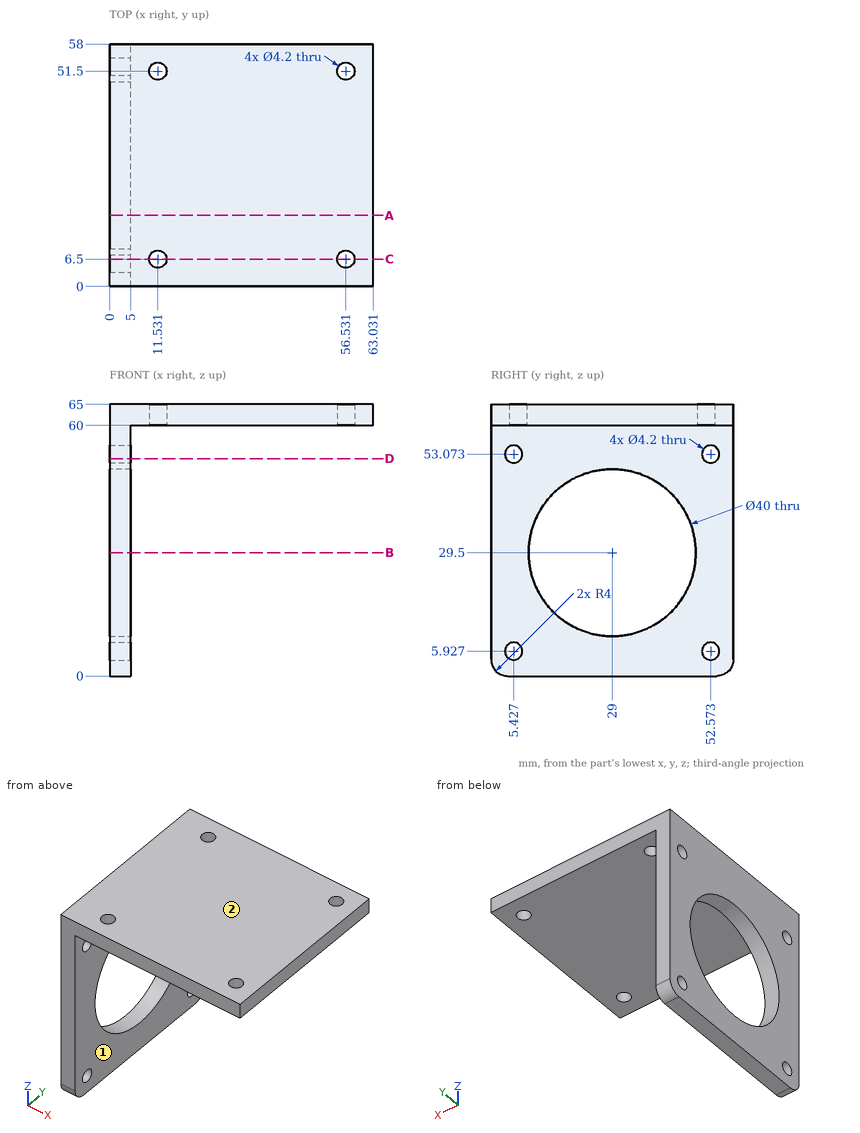
Verification items for this drawing (mm, ordinates from the low corner). A direction names the side the tool comes from. Round coordinates to 2 decimals unless told otherwise and drop trailing zeros. Write each loop counter-clockwise with the first axis right and the second up, starting at its lowest first coordinate (ties: lowest second). Pieces come first, ordered by that corner, then holes. Notation, with made-up numbers: M 24,65 L 50,65 A17 ccw 50,85 Z; hole C 76.25,60 d1. An arc over 180 degrees is marked long. Write item = value, one per line. Start each with the question number.
1. Section check D-D, the plane z = 52. Record the cut outline in (x, y), then the cut area to 3 significant figures.
2. Section check A-A, the plane y = 17. Record the cut outline in (x, z).
3. Section check B-B, the plane z = 29.5. Record the cut outline in (x, y), then the cut area to 3 significant figures.
4. Gauge pin test, flat ends, axial feed: pin 1 (2.5 mm diameter, centred on x = 56.53, y = 51.5, fed in from -Z); pin 2 (5.5 mm diameter, centred on x = 11.53, y = 51.5, fed in from -Z); pin 3 (1 mm diameter, centred on y = 16.5, z = 11, fed in from +X); pin 4 (5 mm diameter, centred on y = 5.43, z = 5.93, fed in from -X). Record the tip position at first contact, or that the pin passes through.
5. Section check C-C, the plane y = 6.5. Record the cut outline in (x, z), then the cut area to 3 significant figures.
6. Scan lines: line 1 (Z direction, x = 46, y = 31.5); line 2 (X direction, y = 18.5, z = 53); line 3 (Z direction, x = 2, y = 29). Record each from-to range of solid material in increasing order. Write a range as [from, to].
7. Tool access check on the marked faces 1 and 2. Record the directions out of +Z, -Z, +X, -X, +Y, -Y that give a thin tool (end or side, any length) a straight path to the whole face; none if there is none.
Results found:
q1.outline = M 0,0 L 5,0 L 5,3.62 L 0,3.62 Z; M 0,7.23 L 5,7.23 L 5,50.77 L 0,50.77 Z; M 0,54.38 L 5,54.38 L 5,58 L 0,58 Z
q1.area = 254 mm^2
q2.outline = M 0,0 L 5,0 L 5,13.5 L 0,13.5 Z; M 0,45.5 L 5,45.5 L 5,60 L 63.03,60 L 63.03,65 L 0,65 Z
q3.outline = M 0,0 L 5,0 L 5,9 L 0,9 Z; M 0,49 L 5,49 L 5,58 L 0,58 Z
q3.area = 90.0 mm^2
q4.pin_1 = through
q4.pin_2 = 60
q4.pin_3 = 5
q4.pin_4 = 0
q5.outline = M 0,0 L 5,0 L 5,4.12 L 0,4.12 Z; M 0,7.73 L 5,7.73 L 5,51.27 L 0,51.27 Z; M 0,54.88 L 5,54.88 L 5,60 L 9.43,60 L 9.43,65 L 0,65 Z; M 13.63,60 L 54.43,60 L 54.43,65 L 13.63,65 Z; M 58.63,60 L 63.03,60 L 63.03,65 L 58.63,65 Z
q5.area = 537 mm^2
q6.line_1 = [60, 65]
q6.line_2 = [0, 5]
q6.line_3 = [0, 9.5], [49.5, 65]
q7.face_1 = -Z, +X, +Y, -Y
q7.face_2 = +Z, +X, -X, +Y, -Y
